The listing builds one solid part. Answer for the finished solid, in the listing's coordinates (mm). A direction names the side the tool comes from. Coordinates: 2 decimals unless noted, no trailing zeros. Order: outer loops, then holes, each group sorted by start corner. A loop starts at its lowest first (then second) coordinate and runs counter-clockwise, first axis right, second up.
Solid Edge part; units mm, degrees
sketch "Sketch1" plane through (0, 0, 0) normal (0, -1, 0) x (1, 0, 0)
  line L0 (50, 37.5) -> (-50, 37.5)
  line L1 (-50, 37.5) -> (-50, -37.5)
  line L2 (-50, -37.5) -> (50, -37.5)
  line L3 (50, -37.5) -> (50, 37.5)
extrude "Protrusion1" add sketch "Sketch1" along normal blind 48
sketch "Sketch2" plane through (0, 0, 0) normal (0, -1, 0) x (1, 0, 0)
  line L0 (14, 12.5) -> (-50, 12.5)
  line L1 (-50, 12.5) -> (-50, -12.5)
  line L2 (-50, -12.5) -> (14, -12.5)
  line L3 (14, -12.5) -> (14, 12.5)
extrude "ExtrudedCutout_2" cut sketch "Sketch2" along normal blind 16
sketch "Sketch3" plane through (0, 0, 0) normal (0, -1, 0) x (1, 0, 0)
  line L0 (-50, -12.5) -> (14, -12.5)
  line L1 (14, -37.5) -> (14, -12.5)
  line L2 (-50, -37.5) -> (14, -37.5)
  line L3 (-50, -12.5) -> (-50, -37.5)
extrude "ExtrudedCutout_3" cut sketch "Sketch3" along normal blind 32
(1) Find section B-B (x = -30). Write down the section's boundary in (y, z), and give its area (3 significant figures).
(2) Find section C-C (z = -16.5). Write down the section's boundary in (x, y).
(3) Each of these flat-tipped pins is pushed along its axis until it touches: pin 1 Ø12.5 at (x, z) = (-29, -3) entering from +Y; pin 2 Ø17.5 at (x, y) = (-23, -22.5) entering from -Z; pin 3 Ø7.5 at (x, z) = (-6, -21.5) entering from +Y. Where does it stop, or does it pass through?
(4) Consider line 1 (X direction, y = -11, z = -34); line 2 (Z direction, x = -3, y = -31); line 3 (Y direction, x = -39.5, z = 5). Determine where each line is inside the solid, lowest interval first.
(5) For faces 1 (the face through (-18, -16, 0)), 2 (the face through (12, 0, 17)), determine the directions among +Z, -Z, +X, -X, +Y, -Y from which every point of the face is accessible in a straight line to the end or side of a thin tool.
(6) Find section A-A (y = -27). Write down the section's boundary in (x, z), and give its area (3 significant figures).
Findings below:
1. outline: (-48, -37.5) - (-32, -37.5) - (-32, -12.5) - (-16, -12.5) - (-16, 12.5) - (0, 12.5) - (0, 37.5) - (-48, 37.5) - close
1. area: 2,400 mm2
2. outline: (-50, -48) - (50, -48) - (50, 0) - (14, 0) - (14, -32) - (-50, -32) - close
3. pin 1: stops at y = -16
3. pin 2: stops at z = -12.5
3. pin 3: stops at y = -32
4. line 1: x = 14 to 50
4. line 2: z = -12.5 to 37.5
4. line 3: y = -48 to -16
5. face 1: -Z, -X, +Y
5. face 2: +Z, -Z, +X, -X, +Y
6. outline: (-50, -12.5) - (14, -12.5) - (14, -37.5) - (50, -37.5) - (50, 37.5) - (-50, 37.5) - close
6. area: 5,900 mm2
